Design review of the part built by this model. Coordinates are the model's own, in mm. A direction names the side the tool comes from. Give positions to 0.01 mm unless a question says otherwise; leave off trailing zeros. Loops run counter-clockwise (first coordinate to the right, second up) from the corner with the lowest first, then second, coordinate; pieces in that order, holes last. Notation, with made-up numbers: (-28.75, -38.75) - (10.25, -38.75) arc R16 ccw to (10.25, -10.75) - close; hole circle Ø1 at (7, 16.25). An arc over 180 degrees is marked (long way). Put each result on its own line as item: value. Start each with the question number.
```python
from build123d import *

# Parameters (mm, degrees)
F1_DEPTH = 15


# Not quite as in the source:
# - ends of sketch curves that miss each other by under 0.0002 mm in the source are joined


with BuildPart() as f1:
    # F0 (on Front) → F1 (new body)
    with BuildSketch(Plane.XZ):
        with BuildLine():
            Line((7.65, 4.781237), (7.250144, 4.781237))
            ThreePointArc((7.250144, 4.781237), (4.0957152155, 1.9799825245), (0, 0.968764))
            ThreePointArc((0, 0.968764), (-4.0957149647, 1.9799823926), (-7.2501430423, 4.7812369709))
            Line((-7.2501430423, 4.7812369709), (-7.65, 4.781237))
            Line((-7.65, 4.781237), (-7.65, -3.681236))
            Line((-7.65, -3.681236), (-5.25, -3.681236))
            Line((-5.25, -3.681236), (-5.25, -4.781236))
            Line((-5.25, -4.781236), (0, -4.781236))
            Line((0, -4.781236), (5.25, -4.781236))
            Line((5.25, -4.781236), (5.25, -3.681236))
            Line((5.25, -3.681236), (7.65, -3.681236))
            Line((7.65, -3.681236), (7.65, 4.781237))
        make_face()
    extrude(amount=F1_DEPTH)


solid = f1.part
```
Item 1: Machinability: for faces 1 (the flat face through (-5.25, -7, -4)), 2 (the flat face through (0, -15, -1)), 3 (the flat face through (6, -7, -3.681)), which of the approach directions +Z, -Z, +X, -X, +Y, -Y give a long, thin tool a straight path to every point of the face, cutting with its end or side? Answer none if there is none.
Item 2: Consider section C-C (z = 2). State the section outline as (x, y) points, plus the area to 3 significant figures.
Item 3: For P1, Ø1.2, axis at x = -6.5, y = -10.5, coming from the -Z side; P2, Ø2, axis at x = -4, y = -12.5, coming from the +Z side, all flat-tipped, find the tip position at first contact; note any pin that passes through.
Item 4: Consider section A-A (y = -7.75). State the section outline as (x, z) points, plus the area to 3 significant figures.
Item 5: Consider section B-B (z = 3.25). State the section outline as (x, y) points.
Item 6: For L1, parallel to Z at x = 0, y = -10; L2, parallel to X at y = -5.75, z = 2.25; L3, parallel to X at y = -3, z = 4.25, list the stretches that pass through material, from the lowest coordinate up. Write a range as from..to.
Item 7: Consider section D-D (x = -6). State the section outline as (y, z) points.
Geometry says:
1. face 1: -Z, -X, +Y, -Y
1. face 2: +Z, -Z, +X, -X, -Y
1. face 3: -Z, +X, +Y, -Y
2. outline: (-7.65, -15) - (-4.13, -15) - (-4.13, 0) - (-7.65, 0) - close; (4.13, -15) - (7.65, -15) - (7.65, 0) - (4.13, 0) - close
2. area: 105 mm2
3. P1: stops at z = -3.68
3. P2: stops at z = 2.53
4. outline: (-7.65, -3.68) - (-5.25, -3.68) - (-5.25, -4.78) - (5.25, -4.78) - (5.25, -3.68) - (7.65, -3.68) - (7.65, 4.78) - (7.25, 4.78) arc R8.8 cw to (0, 0.97) arc R8.8 cw to (-7.25, 4.78) - (-7.65, 4.78) - close
4. area: 102 mm2
5. outline: (-7.65, -15) - (-5.91, -15) - (-5.91, 0) - (-7.65, 0) - close; (5.91, -15) - (7.65, -15) - (7.65, 0) - (5.91, 0) - close
6. L1: z = -4.78..0.97
6. L2: x = -7.65..-4.57, 4.57..7.65
6. L3: x = -7.65..-6.85, 6.85..7.65
7. outline: (-15, -3.68) - (0, -3.68) - (0, 3.33) - (-15, 3.33) - close
